The model under review builds one solid part; all positions refer to its coordinate system, in mm. A direction names the side the tool comes from. Round coordinates to 2 decimals unless told otherwise and drop trailing zeros. Write each loop counter-clockwise with the first axis right and the second up, starting at its lowest first coordinate (ties: lowest second). Pieces come first, ordered by that corner, then holes. Notation, with made-up numbers: (36.25, -27) -> (53.25, -27) arc R9 ccw to (53.25, -13) -> close; hole circle Ø9 at (36, 61). An arc over 180 degrees is marked (long way). Use CSV: the item, a comma, the result in double quotes. Start each with the question number.
1) For pin 1 Ø2 at (x, z) = (23, 0.5) entering from +Y; pin 2 Ø1.6 at (x, z) = (-19, 1) entering from +Y; pin 3 Ø1.6 at (x, z) = (21.5, 1) entering from -Y, all flat-tipped, find the tip position at first contact; note any pin that passes through.
2) Mouldability with a two-part tool opening along X and no side actions: class faces 1 (the face through (31.416, -0.032, 0.986)), 2 (the face through (0, -3, 0)), 3 (the face through (-18, 0.727, 1)) as released by +X, released by -X, zero draft, split by the parting line, or undercut.
3) Wall thickness on probe 1 along X at (y, z) = (-0.25, 4.45); probe 2 along Y at (x, z) = (0, 0.2); probe 3 along Z at (x, y) = (7, 0.5): over which ranges is each line inside the solid? List them lowest first. Write a range as [from, to].
4) Take a section at B-B, the plane z = 4.45. Give the boundary of the cut face in (x, y), then the cut area to 3 significant figures.
5) Take a section at A-A, the plane x = 23. Give the boundary of the cut face in (y, z), then the cut area to 3 significant figures.
6) Machinability: for faces 4 (the face through (13.784, 0.016, 0.986)), 5 (the face through (1, -1, 1)), 6 (the face through (1, -1, 0.5)), 7 (the face through (0, 3, 5)), which of the approach directions +Z, -Z, +X, -X, +Y, -Y give a long, thin tool a straight path to every point of the face, cutting with its end or side? Answer none if there is none.
from build123d import *

# Parameters (mm, degrees)
EXTRUDE_3_DEPTH     = 2
EXTRUDE_3_2_DEPTH   = 2
SKETCH_2_R          = 3.75
SKETCH_2_R_2        = 2.5
EXTRUDE_5_DEPTH     = 3
EXTRUDE_START       = 2
SKETCH_3_R          = 3.75
SKETCH_3_R_2        = 2.5
EXTRUDE_6_DEPTH     = 2
SKETCH_4_R          = 0.5
CUT_EXTRUDE_1_DEPTH = 2
SKETCH_5_R          = 2.5
EXTRUDE_7_DEPTH     = 1
SKETCH_6_R          = 2.5
CUT_EXTRUDE_2_DEPTH = 0.5
SKETCH_7_R          = 1.25
CUT_EXTRUDE_3_DEPTH = 5
CUT_EXTRUDE2_DEPTH  = 2


with BuildPart() as part:
    # Sketch 1 → Extrude 3 (new body)
    with BuildSketch(Plane.XY):
        with BuildLine():
            ThreePointArc((-2.88547071, -2.395111434), (-3.527252129, -1.273182005), (-3.75, 0))
            ThreePointArc((-3.75, 0), (-3.527252129, 1.273182005), (-2.88547071, 2.395111434))
            Line((-2.88547071, 2.395111434), (-29.981181912, 1.434943796))
            ThreePointArc((-29.981181912, 1.434943796), (-31.416125708, 0), (-29.981181912, -1.434943796))
            Line((-29.981181912, -1.434943796), (-2.88547071, -2.395111434))
        make_face()
    extrude(amount=EXTRUDE_3_DEPTH)



with BuildPart() as body_2:
    # Sketch 1 → Extrude 3 2 (new body)
    with BuildSketch(Plane.XY):
        with BuildLine():
            Line((29.981181912, 1.434943796), (2.88547071, 2.395111434))
            ThreePointArc((2.88547071, 2.395111434), (3.75, 0), (2.88547071, -2.395111434))
            Line((2.88547071, -2.395111434), (29.981181912, -1.434943796))
            ThreePointArc((29.981181912, -1.434943796), (31.416125708, 0), (29.981181912, 1.434943796))
        make_face()
    extrude(amount=EXTRUDE_3_2_DEPTH)


with BuildPart() as body_3:
    # Sketch 2 → Extrude 5 (new body)
    with BuildSketch(Plane.XY.offset(2)):
        Circle(SKETCH_2_R)
        Circle(SKETCH_2_R_2, mode=Mode.SUBTRACT)
    extrude(amount=EXTRUDE_5_DEPTH)


with BuildPart() as part_1:
    add(part.part)

    add(body_2.part)  # Extrude 6 merges body 2

    add(body_3.part)  # Extrude 6 merges body 3
    # Sketch 3 → Extrude 6 (add)
    with BuildSketch(Plane(origin=(0, 0, 2), x_dir=(-1, 0, 0), z_dir=(0, 0, -1)).offset(EXTRUDE_START)):
        with Locations(Location((0, 0, 0), (0, 0, 180))):
            Circle(SKETCH_3_R)
        with Locations(Location((0, 0, 0), (0, 0, 180))):
            Circle(SKETCH_3_R_2, mode=Mode.SUBTRACT)
    extrude(amount=-EXTRUDE_6_DEPTH)

    # Sketch 4 → Cut-Extrude 1 (cut)
    with BuildSketch(Plane(origin=(0, 0, 0), x_dir=(-1, 0, 0), z_dir=(0, 0, -1))):
        with Locations((-14.5, 0)):
            Circle(SKETCH_4_R)
        with Locations((-4.5, 0)):
            Circle(SKETCH_4_R)
        with Locations((-6.5, 0)):
            Circle(SKETCH_4_R)
        with Locations((-8.5, 0)):
            Circle(SKETCH_4_R)
        with Locations((-10.5, 0)):
            Circle(SKETCH_4_R)
        with Locations((-12.5, 0)):
            Circle(SKETCH_4_R)
        with Locations((4.5, 0)):
            Circle(SKETCH_4_R)
        with Locations((6.5, 0)):
            Circle(SKETCH_4_R)
        with Locations((8.5, 0)):
            Circle(SKETCH_4_R)
        with Locations((10.5, 0)):
            Circle(SKETCH_4_R)
        with Locations((12.5, 0)):
            Circle(SKETCH_4_R)
        with Locations((14.5, 0)):
            Circle(SKETCH_4_R)
    extrude(amount=-CUT_EXTRUDE_1_DEPTH, mode=Mode.SUBTRACT)

    # Sketch 5 → Extrude 7 (add)
    with BuildSketch(Plane(origin=(0, 0, 0), x_dir=(-1, 0, 0), z_dir=(0, 0, -1))):
        with Locations(Location((0, 0, 0), (0, 0, 180))):
            Circle(SKETCH_5_R)
    extrude(amount=-EXTRUDE_7_DEPTH)

    # Sketch 6 → Cut-Extrude 2 (cut)
    with BuildSketch(Plane(origin=(0, 0, 0), x_dir=(-1, 0, 0), z_dir=(0, 0, -1))):
        with Locations(Location((0, 0, 0), (0, 0, 180))):
            Circle(SKETCH_6_R)
    extrude(amount=-CUT_EXTRUDE_2_DEPTH, mode=Mode.SUBTRACT)

    # Sketch 7 → Cut-Extrude 3 (cut)
    with BuildSketch(Plane(origin=(0, 0, 0.5), x_dir=(-1, 0, 0), z_dir=(0, 0, -1))):
        Circle(SKETCH_7_R)
    extrude(amount=-CUT_EXTRUDE_3_DEPTH, mode=Mode.SUBTRACT)

    # Sketch3 → Cut-Extrude2 (cut)
    with BuildSketch(Plane(origin=(0, 0, 0), x_dir=(-1, 0, 0), z_dir=(0, 0, -1))):
        with BuildLine():
            Line((20.770262951, -0.726731665), (14.5, -0.726731665))
            ThreePointArc((14.5, -0.726731665), (13.773268335, 0), (14.5, 0.726731665))
            Line((14.5, 0.726731665), (20.770262951, 0.726731665))
            ThreePointArc((20.770262951, 0.726731665), (21.496994893, 2.77e-07), (20.770262951, -0.726731665))
        make_face()
        with BuildLine():
            Line((-14.5, -0.716032824), (-30.079105353, -0.716032824))
            ThreePointArc((-30.079105353, -0.716032824), (-30.795138177, 0), (-30.079105353, 0.716032824))
            Line((-30.079105353, 0.716032824), (-14.5, 0.716032824))
            ThreePointArc((-14.5, 0.716032824), (-13.783967176, 0), (-14.5, -0.716032824))
        make_face()
    extrude(amount=-CUT_EXTRUDE2_DEPTH, mode=Mode.SUBTRACT)


solid = part_1.part
Values found:
1,pin 1,"y = 1.72"
1,pin 2,"y = 1.85"
1,pin 3,"y = -1.76"
2,face 1,"released by +X"
2,face 2,"zero draft"
2,face 3,"undercut"
3,probe 1,"[-3.74, -2.49], [2.49, 3.74]"
3,probe 2,"[-3.75, -2.5], [2.5, 3.75]"
3,probe 3,"[0, 2]"
4,outline,"circle Ø7.5 at (0, 0); hole circle Ø5 at (0, 0)"
4,area,"24.5 mm²"
5,outline,"(-1.68, 0) -> (-0.72, 0) -> (-0.72, 2) -> (-1.68, 2) -> close; (0.72, 0) -> (1.68, 0) -> (1.68, 2) -> (0.72, 2) -> close"
5,area,"3.87 mm²"
6,face 4,"+Z, -Z"
6,face 5,"+Z"
6,face 6,"-Z"
6,face 7,"+Z, +X, -X, +Y, -Y"
